Geometry: see drawing. Coordinates: mm, zero at the bounding-box minimum. A direction names the side the tool comes from. Coordinates: 2 decimals unless noted, no trailing zeros. Write each loop counter-clockwise with the first axis right and the second up, starting at its lowest first coordinate (ties: lowest second). Pieces come first, ordered by that corner, then holes. Notation, with made-up numbers: (-12, 38.5) - (9, 38.5) arc R27 ccw to (9, 72.5) - close; hole circle Ø5 at (-10, -7.5). An arc over 180 degrees is marked (long way). Use CSV: the item, a comma, the result in double quotes.
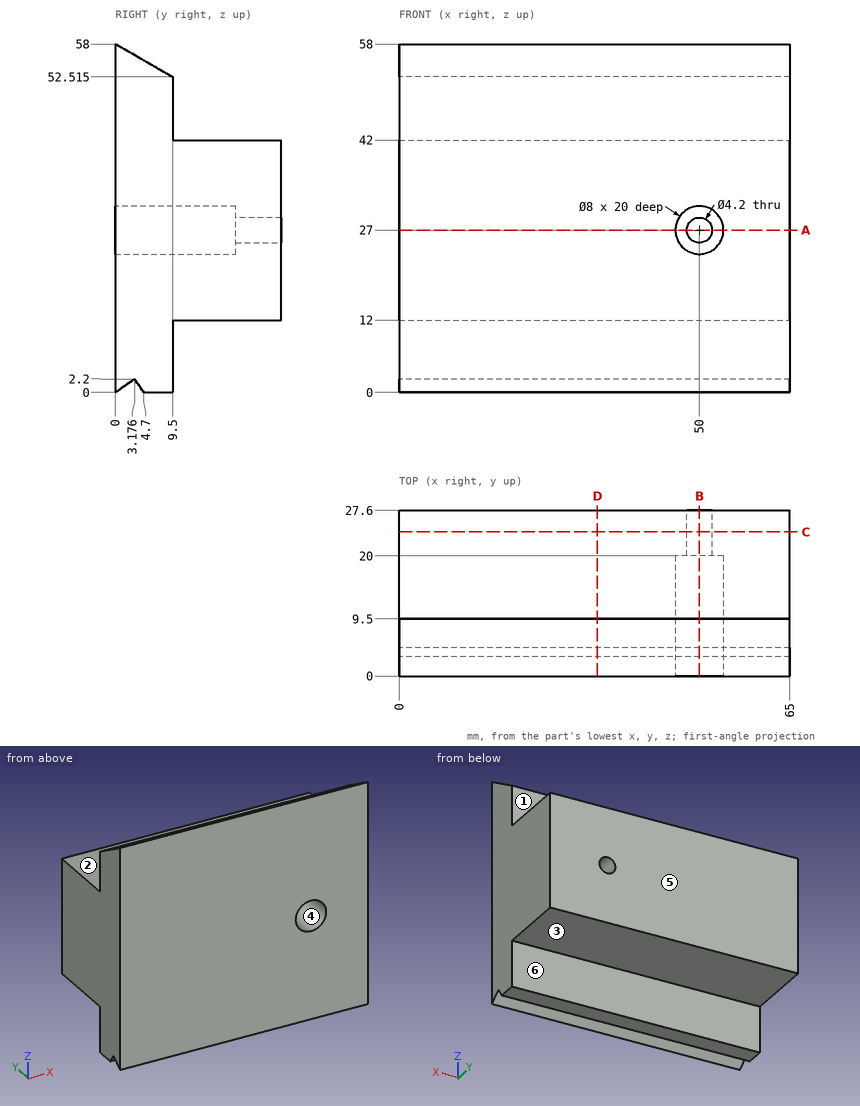
(1) Cut plane C-C on y = 24. Return loops of the section in (x, z), and give its area (3 significant figures).
Check values:
outline,"(0, 12) - (65, 12) - (65, 42) - (0, 42) - close; hole circle Ø4.2 at (50, 27)"
area,"1,940 mm^2"
(2) Draft query along Z for the marked faces 1, 2, 3 and 4. Return one class per face: pulls with the +Z half, pulls with the -Z half, needs draft (parallel to the pull), parting line crosses it, or undercut.
Check values:
face 1,"needs draft"
face 2,"pulls with the +Z half"
face 3,"pulls with the -Z half"
face 4,"undercut"
(3) Ray query, probe 1 along X at (y, z) = (23, 27); probe 2 along X at (y, z) = (12.25, 27); probe 3 along Y at (x, z) = (14.5, 45). Return the intervals inside material, ascending. Write a range as from..to.
Check values:
probe 1,"0..47.9, 52.1..65"
probe 2,"0..46, 54..65"
probe 3,"0..9.5"
(4) Cut plane B-B on x = 50. Return loops of the section in (y, z) (1 decimal).
Check values:
outline,"(0, 0) - (3.2, 2.2) - (4.7, 0) - (9.5, 0) - (9.5, 12) - (27.6, 12) - (27.6, 24.9) - (20, 24.9) - (20, 23) - (0, 23) - close; (0, 31) - (20, 31) - (20, 29.1) - (27.6, 29.1) - (27.6, 42) - (9.5, 42) - (9.5, 52.5) - (0, 58) - close"
(5) Reachability of the marked faces 5 and 6 from +Z, -Z, +X, -X, +Y, -Y: full face, straight path, thin tool, end or side. Return the list, or none.
Check values:
face 5,"+Z, -Z, +X, -X, +Y"
face 6,"-Z, +X, -X, +Y"
(6) Pin query (flat end, axial travel): pin 1 Ø6 at (x, y) = (54.5, 17.5) entering from +Z; pin 2 Ø10 at (x, y) = (14.5, 10) entering from +Z; pin 3 Ø6.5 at (x, z) = (50, 27) entering from -Y. Return the tip coordinate at first contact, or that it passes through.
Check values:
pin 1,"z = 42"
pin 2,"z = 55.11"
pin 3,"y = 20"
(7) Cut plane D-D on x = 33. Return loops of the section in (y, z) (1 decimal), and give its area (3 significant figures).
Check values:
outline,"(0, 0) - (3.2, 2.2) - (4.7, 0) - (9.5, 0) - (9.5, 12) - (27.6, 12) - (27.6, 42) - (9.5, 42) - (9.5, 52.5) - (0, 58) - close"
area,"1,060 mm^2"
(8) Cut plane A-A on z = 27. Return loops of the section in (x, y), and give its area (3 significant figures).
Check values:
outline,"(0, 0) - (46, 0) - (46, 20) - (47.9, 20) - (47.9, 27.6) - (0, 27.6) - close; (52.1, 20) - (54, 20) - (54, 0) - (65, 0) - (65, 27.6) - (52.1, 27.6) - close"
area,"1,600 mm^2"
